Work out the finished part from the listing and answer in its coordinate system (mm). A direction names the side the tool comes from. Round coordinates to 2 decimals unless told otherwise and drop trailing zeros. Write each loop counter-clockwise with the first axis right and the second up, starting at its lowest first coordinate (ties: lowest second). Pieces come first, ordered by that corner, then holes. Notation, with made-up numbers: (-14, 86.5) -> (26, 86.5) arc R14 ccw to (26, 90.5) -> close; hole circle Ø2 at (18, 30.5). An arc over 180 degrees is marked (long way). One line per item, written item: value.
```python
from build123d import *

# Parameters (mm, degrees)
F1_DEPTH = 120
F3_DEPTH = 5
F4_DEPTH = 5
F6_DEPTH = 70
F7_R     = 5
F8_R     = 1
F9_ANGLE = 90


with BuildPart() as f1:
    # F0 (on Right) → F1 (new body)
    with BuildSketch(Plane.YZ):
        with BuildLine():
            Line((-18.2393755255, 0), (0, 0))
            Line((0, 0), (1.3614935385, 3))
            Line((1.3614935385, 3), (25.6223567947, 56.4579031871))
            Line((25.6223567947, 56.4579031871), (20.1315400534, 56.4579031871))
            Line((20.1315400534, 56.4579031871), (-0.5316509101, 10.9273361007))
            ThreePointArc((-0.5316509101, 10.9273361007), (-6.9059303022, 6.8201828356), (-13.2802096943, 10.9273361007))
            Line((-13.2802096943, 10.9273361007), (-18.2393755255, 0))
        make_face()
        Polygon((1.3614935385, 3), (0, 0), (30, 0), (30, 3), align=None)
    extrude(amount=F1_DEPTH)

    # F0 (on Right) + F2 (on Right) → F3 (join)
    with BuildSketch(Plane.YZ):
        with BuildLine():
            Line((-18.2393755255, 0), (0, 0))
            Line((0, 0), (1.3614935385, 3))
            Line((1.3614935385, 3), (25.6223567947, 56.4579031871))
            Line((25.6223567947, 56.4579031871), (20.1315400534, 56.4579031871))
            Line((20.1315400534, 56.4579031871), (-0.5316509101, 10.9273361007))
            ThreePointArc((-0.5316509101, 10.9273361007), (-6.9059303022, 6.8201828356), (-13.2802096943, 10.9273361007))
            Line((-13.2802096943, 10.9273361007), (-18.2393755255, 0))
        make_face()
    with BuildSketch(Plane.YZ):
        Polygon((0, 0), (25.6223567947, 56.4579031871), (7.3829812692, 56.4579031871), (-13.2802096943, 10.9273361007), (-18.2393755255, 0), align=None)
        Polygon((11.2028951482, 40.4136113624), (6.1610765531, 29.3041529933), (0.6974085027, 31.7837359089), (5.7392270978, 42.893194278), align=None, mode=Mode.SUBTRACT)
    extrude(amount=-F3_DEPTH)

    # F0 (on Right) → F4 (join, through all)
    with BuildSketch(Plane.YZ):
        Polygon((1.3614935385, 3), (0, 0), (30, 0), (30, 3), align=None)
    extrude(amount=-F4_DEPTH)

    # F5 (on face) → F6 (cut)
    with BuildSketch(Plane.YZ.offset(120)):
        with BuildLine():
            ThreePointArc((-9.3360822182, 7.2555532448), (-10.7003955127, 7.9378334949), (-11.8845214943, 8.8994481606))
            Line((-11.8845214943, 8.8994481606), (-12.4811800626, 7.5847333608))
            Line((-12.4811800626, 7.5847333608), (-9.7493460374, 6.344941903))
            Line((-9.7493460374, 6.344941903), (-9.3360822182, 7.2555532448))
        make_face()
        Polygon((14.3532357317, 43.7256261138), (6.5012231655, 26.424010621), (7.4118345073, 26.0107468017), (15.2638470734, 43.3123622945), align=None)
    extrude(amount=-F6_DEPTH, mode=Mode.SUBTRACT)

    # F7 (call 1 of 4: OpenCascade refuses the feature's edges together)
    f7_edges = [f1.edges().sort_by_distance(p)[0] for p in [
        (57.5, -18.239376, 0),
    ]]
    fillet(f7_edges, radius=F7_R)

    # F7#2 (call 2 of 4)
    f7_2_edges = [f1.edges().sort_by_distance(p)[0] for p in [
        (-2.5, 7.382981, 56.457903),
    ]]
    fillet(f7_2_edges, radius=F7_R)

    # F7#4 (call 3 of 4)
    f7_4_edges = [f1.edges().sort_by_distance(p)[0] for p in [
        (57.5, 1.361494, 3),
    ]]
    fillet(f7_4_edges, radius=F7_R)

    # F7#3 (call 4 of 4)
    f7_3_edges = [f1.edges().sort_by_distance(p)[0] for p in [
        (57.5, 25.622357, 56.457903),
    ]]
    fillet(f7_3_edges, radius=F7_R)

    # F8
    f8_edges = [f1.edges().sort_by_distance(p)[0] for p in [
        (57.5, 30, 3),
        (57.5, 30, 0),
    ]]
    fillet(f8_edges, radius=F8_R)


with BuildPart() as f1_1:
    # F9: moved
    add(f1.part.rotate(Axis((-5, 9.2602985566, 0), (0, -1, 0)), F9_ANGLE))


solid = f1_1.part
```
(1) Find section C-C on x = -25. Give the vertices of the cut face in (y, z).
Reported:
outline: (-9.16, 0) -> (9.08, 0) -> (9.08, 125) -> (3.59, 125) -> (3.59, 5) -> (-9.16, 5) -> close
(2) Find section D-D on y = -5. Give the vertices of the cut face in (x, z).
Reported:
outline: (-34.17, 0) -> (-5, 0) -> (-5, 125) -> (-12.08, 125) -> (-12.08, 5) -> (-34.17, 5) -> close
(3) Find section A-A on z = 45. Give the vertices of the cut face in (x, y).
Reported:
outline: (-61.01, 19.93) -> (-15.93, -0.53) arc R7 cw to (-15.93, -13.28) -> (-12.07, -15.03) arc R5 ccw to (-5, -10.48) -> (-5, 29) arc R1 ccw to (-6, 30) -> (-7, 30) arc R1 ccw to (-8, 29) -> (-8, 9.12) arc R5 cw to (-15.07, 4.57) -> (-54.39, 22.42) arc R5 ccw to start
(4) For a pull along X with two mould halves and no side action, classify faces 1 (the face through (-21, 5, 125)), 2 (the face through (-10.35, 4.88, 63.38)), 3 (the face through (-46.67, 8.43, 2.54)), 4 (the face through (-5, 9, 63)) as pulls with the +X half, pulls with the -X half, needs draft (parallel to the pull), parting line crosses it, or undercut.
Reported:
face 1: needs draft
face 2: undercut
face 3: undercut
face 4: pulls with the +X half
(5) Find section B-B on x = -42. Give the vertices of the cut face in (y, z).
Reported:
outline: (-1.45, 0) -> (3.06, 0) -> (3.06, 5) -> (-1.45, 5) -> close; (9.65, 0) -> (16.79, 0) -> (16.79, 125) -> (12.4, 125) -> (12.4, 55) -> (11.3, 55) -> (11.3, 5) -> (9.65, 5) -> close
(6) Flat-ended cylindrical pins translate along their axes: pin 1 Ø2 at (x, z) = (-32.5, 110.5) entering from +Y; pin 2 Ø10 at (y, z) = (19.5, 31.5) entering from -X; pin 3 Ø4 at (x, z) = (-29.5, 97.5) entering from +Y. Find the tip coordinate at first contact, or state that the pin passes through.
Reported:
pin 1: stops at y = 12.93
pin 2: stops at x = -61.01
pin 3: stops at y = 12.03
(7) A tool of negligible diameter and unlimited length cuts with its end or side. For faces 5 (the face through (-60.683, 7.93, 2.465)), 6 (the face through (-38.78, 9.84, 50.83)), 7 (the face through (-34.454, 13.367, 63.375)), 8 (the face through (-11.97, -11.13, 90.49)), 9 (the face through (-35.527, 3.467, 2.535)), from which of +Z, -Z, +X, -X, +Y, -Y can it reach the whole face along a straight path? Write none if from no direction.
Reported:
face 5: +Z, -Z, -X, -Y
face 6: +Z, -X, -Y
face 7: +Z, -Z, +Y
face 8: +Z
face 9: +Z, -Z
(8) Consider probe 1 along Z at (x, y) = (-44, 3.5); probe 2 along X at (y, z) = (-1, 100); probe 3 along X at (y, z) = (-6.5, 86). Determine where each line is inside the solid, lowest interval first.
Reported:
probe 1: z = 0 to 5
probe 2: x = -15.06 to -5
probe 3: x = -11.83 to -5
